Input: part model. Units: mm. Frame: model coordinates. Face numbers are marked on the shaded views. A direction names the side the tool comes from. Coordinates: 2 decimals unless noted, no trailing zeros. Write each loop counter-clockwise with the first axis right and the second up, starting at its lowest first coordinate (ties: lowest second). Pieces come first, ordered by that corner, then holes. Notation, with made-up numbers: (12.5, -25) - (50.5, -25) arc R14 ccw to (50.5, -13) - close; hole circle Ø8 at (-3.75, 29). An arc over 180 degrees is marked (long way). Put each result on its own line as item: value. Start each with the question number.
1. Pull-direction query (X, two-part tool) for the marked faces 1, 2 and 3; classes: released by +X, released by -X, zero draft, split by the parting line, or undercut.
2. Cut plane C-C, the plane y = -5. Return loops of the section in (x, z) (3 decimals).
3. Pin query (flat end, axial travel): pin 1 (6 mm diameter, centred on y = 16.5, z = 42.5, fed in from +X); pin 2 (13 mm diameter, centred on x = 4, y = 52.5, fed in from +Z); pin 3 (3 mm diameter, centred on x = 6.5, z = 16.5, fed in from +Y); pin 4 (17.5 mm diameter, centred on x = 21.5, y = 6, fed in from +Z). Return the tip coordinate at first contact, or that it passes through.
4. Cut plane D-D, the plane z = 54. Return loops of the section in (x, y), and give its area (3 significant figures).
5. Cut plane B-B, the plane y = 22. Return loops of the section in (x, z), and give its area (3 significant figures).
6. Cut plane A-A, the plane x = 20. Return loops of the section in (y, z), and give its area (3 significant figures).
7. Line query: line 1 (Y direction, x = 34, z = 20); line 2 (X direction, y = 23.25, z = 60); line 3 (Y direction, x = 20, z = 7.25). Output: solid intervals per line, ascending.
8. Access query for the marked faces 4, 5, 6, 7 and 8. Directions: +Z, -Z, +X, -X, +Y, -Y. A direction counts if a zero-diameter tool reaches every point of the face in a straight line with its end or side. Return the directions, or none.
from build123d import *

# Parameters (mm, degrees)
SKETCH1_R           = 8
BOSS_EXTRUDE1_DEPTH = 12
SKETCH2_R           = 8
BOSS_EXTRUDE2_DEPTH = 12
SKETCH3_W           = 12
SKETCH3_H           = 48
BOSS_EXTRUDE3_DEPTH = 40
SKETCH4_R           = 8
CUT_EXTRUDE1_DEPTH  = 40
FILLET1_R           = 5


with BuildPart() as part:
    # Sketch1 → Boss-Extrude1 (new body)
    with BuildSketch(Plane.XY):
        with BuildLine():
            Line((0, 0), (0, 20))
            Line((0, 20), (40, 20))
            Line((40, 20), (40, 0))
            ThreePointArc((40, 0), (20, -20), (0, 0))
        make_face()
        with Locations((20, 0)):
            Circle(SKETCH1_R, mode=Mode.SUBTRACT)
    extrude(amount=BOSS_EXTRUDE1_DEPTH)

    # Sketch2 → Boss-Extrude2 (add)
    with BuildSketch(Plane(origin=(0, 20, 0), x_dir=(1, 0, 0), z_dir=(0, 1, 0))):
        with BuildLine():
            Line((0, 0), (40, 0))
            Line((40, 0), (40, -60))
            ThreePointArc((40, -60), (20, -80), (0, -60))
            Line((0, -60), (0, 0))
        make_face()
        with Locations(Location((20, -60, 0), (0, 0, 270))):
            Circle(SKETCH2_R, mode=Mode.SUBTRACT)
    extrude(amount=BOSS_EXTRUDE2_DEPTH)

    # Sketch3 → Boss-Extrude3 (add)
    with BuildSketch(Plane(origin=(0, 0, 0), x_dir=(-1, 0, 0), z_dir=(0, 0, -1))):
        with Locations((-34, 56)):
            Rectangle(SKETCH3_W, SKETCH3_H)
        with Locations((-6, 56)):
            Rectangle(SKETCH3_W, SKETCH3_H)
    extrude(amount=-BOSS_EXTRUDE3_DEPTH)

    # Sketch4 → Cut-Extrude1 (cut)
    with BuildSketch(Plane(origin=(40, 0, 0), x_dir=(0, 0, -1), z_dir=(1, 0, 0))):
        with BuildLine():
            ThreePointArc((-20, 80), (-5.857864376, 74.142135624), (0, 60))
            Line((0, 60), (0, 80))
            Line((0, 80), (-20, 80))
        make_face()
        with BuildLine():
            ThreePointArc((-40, 60), (-34.142135624, 74.142135624), (-20, 80))
            Line((-20, 80), (-40, 80))
            Line((-40, 80), (-40, 60))
        make_face()
        with Locations((-20, 60)):
            Circle(SKETCH4_R)
    extrude(amount=-CUT_EXTRUDE1_DEPTH, mode=Mode.SUBTRACT)

    # Fillet1
    fillet1_edges = [part.edges().sort_by_distance(p)[0] for p in [
        (20, 20, 12),
        (34, 32, 40),
        (6, 32, 40),
    ]]
    fillet(fillet1_edges, radius=FILLET1_R)


solid = part.part
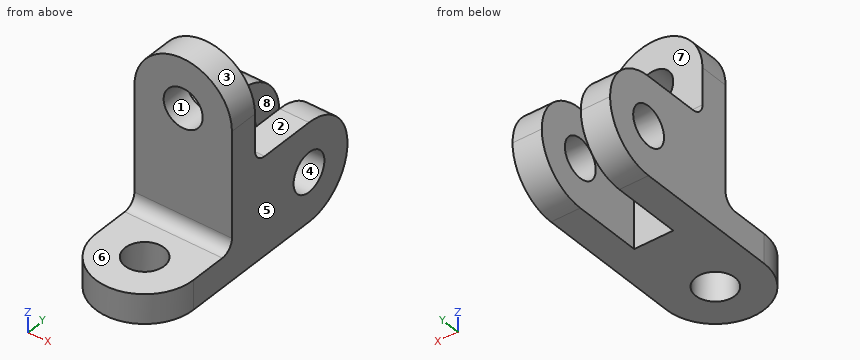
Report:
1. face 1: undercut
1. face 2: zero draft
1. face 3: split by the parting line
2. outline: (0.635, 0) - (13.755, 0) - (13.755, 12) - (0.635, 12) - close; (26.245, 0) - (39.365, 0) - (39.365, 12) - (26.245, 12) - close
3. pin 1: passes through
3. pin 2: stops at z = 40
3. pin 3: stops at y = 79.9
3. pin 4: stops at z = 12
4. outline: (0, 20) - (14.71, 20) - (14.71, 32) - (0, 32) - close; (25.29, 20) - (40, 20) - (40, 32) - (25.29, 32) - close
4. area: 353 mm^2
5. outline: (0, 0) - (40, 0) - (40, 60) arc R20 ccw to (0, 60) - close; hole circle Ø16 at (20, 60)
5. area: 2,830 mm^2
6. outline: (-20, 0) - (-8, 0) - (-8, 12) - (-20, 12) - close; (8, 0) - (32, 0) - (32, 52) - (20, 52) - (20, 17) arc R5 cw to (15, 12) - (8, 12) - close; (20, 68) - (32, 68) - (32, 80) - (20, 80) - close
6. area: 1,060 mm^2
7. line 1: y = 20 to 52, 68 to 80
7. line 2: x = 0 to 12, 28 to 40
7. line 3: y = -20 to -8, 8 to 32
8. face 4: +X, -X
8. face 5: +Z, -Z, +X, +Y, -Y
8. face 6: +Z, +X, -X, -Y
8. face 7: +Z, +Y
8. face 8: +Z, -Z, +Y
